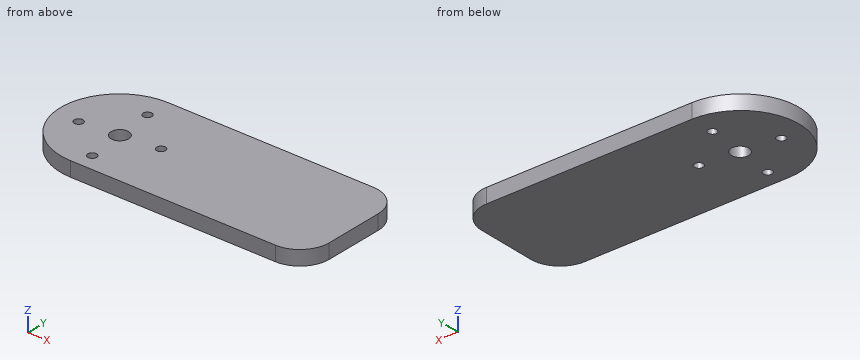
```python
from build123d import *

# Parameters (mm, degrees)
SKETCH1_R           = 1.5
BOSS_EXTRUDE1_DEPTH = 5
SKETCH2_R           = 3
CUT_EXTRUDE1_DEPTH  = 10
FILLET1_R           = 10


with BuildPart() as part:
    # Sketch1 → Boss-Extrude1 (new body)
    with BuildSketch(Plane.XY):
        with BuildLine():
            Line((0, 20), (80, 20))
            Line((80, 20), (80, -20))
            Line((80, -20), (0, -20))
            ThreePointArc((0, -20), (-20, 0), (0, 20))
        make_face()
        with Locations((0, 11.564458964)):
            Circle(SKETCH1_R, mode=Mode.SUBTRACT)
        with Locations((14.292070839, 0)):
            Circle(SKETCH1_R, mode=Mode.SUBTRACT)
        with Locations((2.727611874, -14.292070839)):
            Circle(SKETCH1_R, mode=Mode.SUBTRACT)
        with Locations((-11.564458964, -2.727611874)):
            Circle(SKETCH1_R, mode=Mode.SUBTRACT)
    extrude(amount=BOSS_EXTRUDE1_DEPTH)

    # Sketch2 → Cut-Extrude1 (cut)
    with BuildSketch(Plane(origin=(0, 0, 0), x_dir=(-1, 0, 0), z_dir=(0, 0, -1))):
        with Locations((-1.363805937, -1.363805937)):
            Circle(SKETCH2_R)
    extrude(amount=-CUT_EXTRUDE1_DEPTH, mode=Mode.SUBTRACT)

    # Fillet1
    fillet1_edges = [part.edges().sort_by_distance(p)[0] for p in [
        (80, 20, 2.5),
        (80, -20, 2.5),
    ]]
    fillet(fillet1_edges, radius=FILLET1_R)


solid = part.part
```
Could you check a few things on this model? Use its own coordinates, in mm. Coordinates: 2 decimals unless noted, no trailing zeros. Loops run counter-clockwise (first coordinate to the right, second up) from the corner with the lowest first, then second, coordinate; pieces in that order, holes last.
1) Please list where these lines run through material, in increasing order: line 1 along X through (y, z) = (-2, 3.25); line 2 along X through (y, z) = (11, 3.95); line 3 along Y through (x, z) = (-11, 1.1).
Reported:
line 1: x = -19.9 to -12.88, -10.25 to -1.57, 4.3 to 80
line 2: x = -16.7 to -1.39, 1.39 to 79.95
line 3: y = -16.7 to -4.12, -1.34 to 16.7
2) Imagine slicing it at C-C (x = 74.5). List the corners of the cut face in (y, z) for me, and give its area (3 significant figures).
Reported:
outline: (-18.93, 0) - (18.93, 0) - (18.93, 5) - (-18.93, 5) - close
area: 189 mm2
3) Imagine slicing it at B-B (y = 0). List the corners of the cut face in (x, z) for me.
Reported:
outline: (-20, 0) - (-1.31, 0) - (-1.31, 5) - (-20, 5) - close; (4.04, 0) - (12.79, 0) - (12.79, 5) - (4.04, 5) - close; (15.79, 0) - (80, 0) - (80, 5) - (15.79, 5) - close
4) Imagine slicing it at A-A (z = 2.05). List the corners of the cut face in (x, y) for me, and give its area (3 significant figures).
Reported:
outline: (0, -20) - (70, -20) arc R10 ccw to (80, -10) - (80, 10) arc R10 ccw to (70, 20) - (0, 20) arc R20 ccw to start; hole circle Ø3 at (-11.56, -2.73); hole circle Ø6 at (1.36, -1.36); hole circle Ø3 at (0, 11.56); hole circle Ø3 at (2.73, -14.29); hole circle Ø3 at (14.29, 0)
area: 3,730 mm2
